Could you check a few things on this model? Use its own coordinates, in mm. Face numbers are marked on the shaded views. Coordinates: 2 decimals unless noted, no trailing zeros. Write each loop counter-clockwise with the first axis right and the second up, starting at its lowest first coordinate (ties: lowest second). Pieces come first, ordered by that corner, then holes.
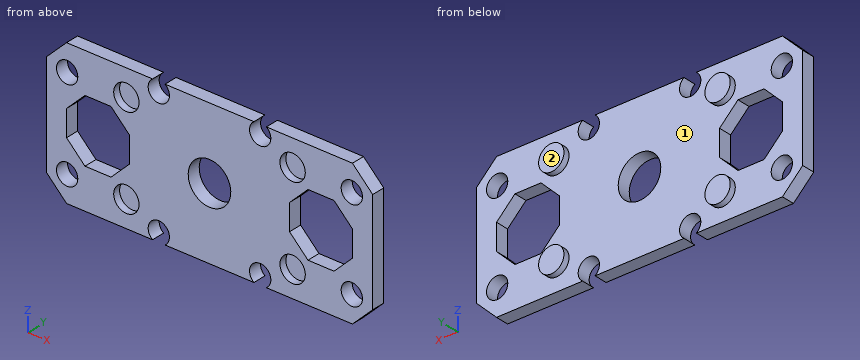
```python
from build123d import *

# Parameters (mm, degrees)
SKETCH1_R           = 1.3335
SKETCH1_R_2         = 1.5875
BOSS_EXTRUDE1_DEPTH = 1.651
CHAMFER1_SIZE       = 2.54
SKETCH1_2_R         = 1.5875
BOSS_EXTRUDE2_DEPTH = 2.413
SKETCH1_3_R         = 1.5875
CUT_EXTRUDE1_DEPTH  = 0.889
SKETCH3_R           = 2.667
CUT_EXTRUDE3_DEPTH  = 23.382376376


with BuildPart() as part:
    # Sketch1 → Boss-Extrude1 (new body)
    with BuildSketch(Plane(origin=(0, 0, 0), x_dir=(1, 0, 0), z_dir=(0, 1, 0))):
        with BuildLine():
            Line((-5.567119422, 8.9535), (5.567119422, 8.9535))
            ThreePointArc((5.567119422, 8.9535), (6.35, 6.5405), (7.132880578, 8.9535))
            Line((7.132880578, 8.9535), (20.447, 8.9535))
            Line((20.447, 8.9535), (20.447, -8.9535))
            Line((20.447, -8.9535), (7.132880578, -8.9535))
            ThreePointArc((7.132880578, -8.9535), (6.35, -6.5405), (5.567119422, -8.9535))
            Line((5.567119422, -8.9535), (-5.567119422, -8.9535))
            ThreePointArc((-5.567119422, -8.9535), (-6.35, -6.5405), (-7.132880578, -8.9535))
            Line((-7.132880578, -8.9535), (-20.447, -8.9535))
            Line((-20.447, -8.9535), (-20.447, 8.9535))
            Line((-20.447, 8.9535), (-7.132880578, 8.9535))
            ThreePointArc((-7.132880578, 8.9535), (-6.35, 6.5405), (-5.567119422, 8.9535))
        make_face()
        with Locations(Location((-17.8308, 5.6769, 0), (0, 0, 90))):
            Circle(SKETCH1_R, mode=Mode.SUBTRACT)
        with Locations(Location((17.8308, 5.6769, 0), (0, 0, 90))):
            Circle(SKETCH1_R, mode=Mode.SUBTRACT)
        with Locations(Location((17.8308, -5.6769, 0), (0, 0, 90))):
            Circle(SKETCH1_R, mode=Mode.SUBTRACT)
        with Locations(Location((-17.8308, -5.6769, 0), (0, 0, 90))):
            Circle(SKETCH1_R, mode=Mode.SUBTRACT)
        with Locations(Location((-10.414, 5.6769, 0), (0, 0, 90))):
            Circle(SKETCH1_R_2, mode=Mode.SUBTRACT)
        with Locations(Location((10.414, 5.6769, 0), (0, 0, 90))):
            Circle(SKETCH1_R_2, mode=Mode.SUBTRACT)
        with Locations(Location((10.414, -5.6769, 0), (0, 0, 90))):
            Circle(SKETCH1_R_2, mode=Mode.SUBTRACT)
        with Locations(Location((-10.414, -5.6769, 0), (0, 0, 90))):
            Circle(SKETCH1_R_2, mode=Mode.SUBTRACT)
    extrude(amount=BOSS_EXTRUDE1_DEPTH)

    # Chamfer1
    chamfer1_edges = [part.edges().sort_by_distance(p)[0] for p in [
        (20.447, 0.8255, -8.9535),
        (20.447, 0.8255, 8.9535),
        (-20.447, 0.8255, 8.9535),
        (-20.447, 0.8255, -8.9535),
    ]]
    chamfer(chamfer1_edges, length=CHAMFER1_SIZE)

    # Sketch1_2 → Boss-Extrude2 (add)
    with BuildSketch(Plane(origin=(0, 0, 0), x_dir=(1, 0, 0), z_dir=(0, 1, 0))):
        with Locations(Location((-10.414, 5.6769, 0), (0, 0, 270))):
            Circle(SKETCH1_2_R)
        with Locations(Location((10.414, 5.6769, 0), (0, 0, 270))):
            Circle(SKETCH1_2_R)
        with Locations(Location((10.414, -5.6769, 0), (0, 0, 270))):
            Circle(SKETCH1_2_R)
        with Locations(Location((-10.414, -5.6769, 0), (0, 0, 270))):
            Circle(SKETCH1_2_R)
    extrude(amount=BOSS_EXTRUDE2_DEPTH)

    # Sketch1_3 → Cut-Extrude1 (cut)
    with BuildSketch(Plane(origin=(0, 0, 0), x_dir=(1, 0, 0), z_dir=(0, 1, 0))):
        with Locations(Location((-10.414, 5.6769, 0), (0, 0, 270))):
            Circle(SKETCH1_3_R)
        with Locations(Location((10.414, 5.6769, 0), (0, 0, 270))):
            Circle(SKETCH1_3_R)
        with Locations(Location((10.414, -5.6769, 0), (0, 0, 270))):
            Circle(SKETCH1_3_R)
        with Locations(Location((-10.414, -5.6769, 0), (0, 0, 270))):
            Circle(SKETCH1_3_R)
    extrude(amount=CUT_EXTRUDE1_DEPTH, mode=Mode.SUBTRACT)

    # Sketch3 → Cut-Extrude3 (cut, through all)
    with BuildSketch(Plane(origin=(0, 1.651, 0), x_dir=(1, 0, 0), z_dir=(0, 1, 0))):
        with Locations(Location((0, 0, 0), (0, 0, 270))):
            Circle(SKETCH3_R)
        Polygon((-10.033, 1.630758795), (-12.339241205, 3.937), (-15.600758795, 3.937), (-17.907, 1.630758795), (-17.907, -1.630758795), (-15.600758795, -3.937), (-12.339241205, -3.937), (-10.033, -1.630758795), align=None)
        Polygon((17.907, 1.630758795), (15.600758795, 3.937), (12.339241205, 3.937), (10.033, 1.630758795), (10.033, -1.630758795), (12.339241205, -3.937), (15.600758795, -3.937), (17.907, -1.630758795), align=None)
    extrude(amount=-CUT_EXTRUDE3_DEPTH, mode=Mode.SUBTRACT)


solid = part.part
```
1. I want a section at A-A on x = 13. Please give me the cut outline in (y, z).
Verdict:
outline: (0, -8.95) - (1.65, -8.95) - (1.65, -3.94) - (0, -3.94) - close; (0, 3.94) - (1.65, 3.94) - (1.65, 8.95) - (0, 8.95) - close
2. Please list where these lines run through material, in increasing order: line 1 along X through (y, z) = (1.6, 7.5); line 2 along Z through (x, y) = (-10, 0.15); line 3 along X through (y, z) = (0.15, 2).
Verdict:
line 1: x = -19.36 to -7.63, -5.07 to 5.07, 7.63 to 19.36
line 2: z = -8.95 to -7.21, -4.14 to 4.14, 7.21 to 8.95
line 3: x = -20.45 to -17.54, -10.4 to -1.76, 1.76 to 10.4, 17.54 to 20.45
3. I want a section at B-B on z = 0. Please give me the cut outline in (x, y).
Verdict:
outline: (-20.45, 0) - (-17.91, 0) - (-17.91, 1.65) - (-20.45, 1.65) - close; (-10.03, 0) - (-2.67, 0) - (-2.67, 1.65) - (-10.03, 1.65) - close; (2.67, 0) - (10.03, 0) - (10.03, 1.65) - (2.67, 1.65) - close; (17.91, 0) - (20.45, 0) - (20.45, 1.65) - (17.91, 1.65) - close
4. I want a section at C-C on z = -3.25. Please give me the cut outline in (x, y).
Verdict:
outline: (-20.45, 0) - (-16.29, 0) - (-16.29, 1.65) - (-20.45, 1.65) - close; (-11.65, 0) - (11.65, 0) - (11.65, 1.65) - (-11.65, 1.65) - close; (16.29, 0) - (20.45, 0) - (20.45, 1.65) - (16.29, 1.65) - close
5. If we mould it in two halves opening along X, with no side actions, what happens to the marked faces 1 and 2? For each: pulls with the +X half, pulls with the -X half, needs draft (parallel to the pull), parting line crosses it, or undercut.
Verdict:
face 1: undercut
face 2: needs draft
6. For pin 1 (6 mm diameter, centred on x = -15.5, z = 3.5, fed in from +Y), with a flat end and sliding along its axis, tell me the tip position at first contact or that it passes through.
Verdict:
pin 1: stops at y = 1.65
7. I want a section at D-D on x = -17. Please give me the cut outline in (y, z).
Verdict:
outline: (0, -8.95) - (1.65, -8.95) - (1.65, -6.72) - (0, -6.72) - close; (0, -4.63) - (1.65, -4.63) - (1.65, -2.54) - (0, -2.54) - close; (0, 2.54) - (1.65, 2.54) - (1.65, 4.63) - (0, 4.63) - close; (0, 6.72) - (1.65, 6.72) - (1.65, 8.95) - (0, 8.95) - close
